Could you check a few things on this model? Use its own coordinates, in mm. A direction names the side the tool comes from. Give positions to 0.01 mm unless a question says otherwise; leave off trailing zeros. Order: outer loops, then holes, each group sorted by start corner. A loop starts at its lowest first (then second) coordinate and runs counter-clockwise, first axis right, second up.
(1) Imagine slicing it at A-A, the plane x = -46. Write out the boundary of the cut face in (y, z).
(2) If I drill on probe 1 along Z at (x, y) = (-12, -18.5); probe 2 along Z at (x, y) = (-46.5, -26.5); probe 3 along Y at (x, z) = (-13, -15), over which ranges is the centre line in solid material (lowest first)?
(3) Imagine slicing it at B-B, the plane y = 44. Write out the boundary of the cut face in (x, z).
(4) Imagine slicing it at C-C, the plane z = 3. Write out the boundary of the cut face in (x, y).
(5) Imagine slicing it at D-D, the plane y = -28. Write out the boundary of the cut face in (x, z).
(6) On a 3-axis mill with a long thin cutter (end or side, diameter ignored), from which of +Z, -Z, +X, -X, +Y, -Y can I reach the whole of each face in a straight line? I mean faces 1 (the flat face through (-5, -55, -6.604)), 2 (the flat face through (0, 0, 243.84)), 3 (the flat face through (9.6, 49.2, 0)). Say none if no direction works.
(7) Will these pins go through, and if not, where does the flat tip stop? pin 1 (8 mm diameter, centred on x = -14.5, z = 207.5, fed in from +Y); pin 2 (2 mm diameter, centred on x = -30, y = 31, fed in from +Z); pin 3 (23.5 mm diameter, centred on x = -7, y = -18.5, fed in from +Z).
from build123d import *

# Parameters (mm, degrees)
SKETCH1_R           = 49.9618
BOSS_EXTRUDE1_DEPTH = 78.74
SKETCH2_R           = 66.802
BOSS_EXTRUDE2_DEPTH = 6.604
SKETCH3_R           = 54.864
BOSS_EXTRUDE3_DEPTH = 17.78
SKETCH4_R           = 11.878006526
BOSS_EXTRUDE4_DEPTH = 12.7
BOSS_EXTRUDE5_DEPTH = 38.1
SKETCH7_R           = 39.497
BOSS_EXTRUDE6_DEPTH = 160.02
SKETCH8_R           = 6.058651835
BOSS_EXTRUDE7_DEPTH = 5.08


with BuildPart() as part:
    # Sketch1 → Boss-Extrude1 (new body)
    with BuildSketch(Plane.XY):
        Circle(SKETCH1_R)
    extrude(amount=BOSS_EXTRUDE1_DEPTH)

    # Sketch2 → Boss-Extrude2 (add)
    with BuildSketch(Plane(origin=(0, 0, 0), x_dir=(-1, 0, 0), z_dir=(0, 0, -1))):
        with Locations(Location((0, 0, 0), (0, 0, 180))):
            Circle(SKETCH2_R)
    extrude(amount=BOSS_EXTRUDE2_DEPTH)

    # Sketch3 → Boss-Extrude3 (add)
    with BuildSketch(Plane(origin=(0, 0, -6.604), x_dir=(-1, 0, 0), z_dir=(0, 0, -1))):
        Circle(SKETCH3_R)
    extrude(amount=BOSS_EXTRUDE3_DEPTH)

    # Sketch4 → Boss-Extrude4 (add)
    with BuildSketch(Plane(origin=(0, 0, -24.384), x_dir=(-1, 0, 0), z_dir=(0, 0, -1))):
        Circle(SKETCH4_R)
    extrude(amount=BOSS_EXTRUDE4_DEPTH)

    # Sketch5 → Boss-Extrude5 (add)
    with BuildSketch(Plane(origin=(0, 0, -37.084), x_dir=(-1, 0, 0), z_dir=(0, 0, -1))):
        Polygon((8.315334724, 0), (5.74575498, 1.866908963), (6.727247106, 4.887631119), (3.551071869, 4.887631119), (2.569579744, 7.908353274), (0, 6.041444312), (-2.569579744, 7.908353274), (-3.551071869, 4.887631119), (-6.727247106, 4.887631119), (-5.74575498, 1.866908963), (-8.315334724, 0), (-5.74575498, -1.866908963), (-6.727247106, -4.887631119), (-3.551071869, -4.887631119), (-2.569579744, -7.908353274), (0, -6.041444312), (2.569579744, -7.908353274), (3.551071869, -4.887631119), (6.727247106, -4.887631119), (5.74575498, -1.866908963), align=None)
    extrude(amount=BOSS_EXTRUDE5_DEPTH)

    # Sketch7 → Boss-Extrude6 (add)
    with BuildSketch(Plane.XY.offset(78.74)):
        Circle(SKETCH7_R)
    extrude(amount=BOSS_EXTRUDE6_DEPTH)

    # Sketch8 → Boss-Extrude7 (add)
    with BuildSketch(Plane.XY.offset(238.76)):
        Circle(SKETCH8_R)
    extrude(amount=BOSS_EXTRUDE7_DEPTH)


solid = part.part
Answer block:
1. outline: (-48.44, -6.6) - (-29.9, -6.6) - (-29.9, -24.38) - (29.9, -24.38) - (29.9, -6.6) - (48.44, -6.6) - (48.44, 0) - (19.5, 0) - (19.5, 78.74) - (-19.5, 78.74) - (-19.5, 0) - (-48.44, 0) - close
2. probe 1: z = -24.38 to 238.76
2. probe 2: z = -24.38 to 0
2. probe 3: y = -53.3 to 53.3
3. outline: (-50.26, -6.6) - (-32.77, -6.6) - (-32.77, -24.38) - (32.77, -24.38) - (32.77, -6.6) - (50.26, -6.6) - (50.26, 0) - (23.67, 0) - (23.67, 78.74) - (-23.67, 78.74) - (-23.67, 0) - (-50.26, 0) - close
4. outline: circle Ø99.92 at (0, 0)
5. outline: (-60.65, -6.6) - (-47.18, -6.6) - (-47.18, -24.38) - (47.18, -24.38) - (47.18, -6.6) - (60.65, -6.6) - (60.65, 0) - (41.38, 0) - (41.38, 78.74) - (27.86, 78.74) - (27.86, 238.76) - (-27.86, 238.76) - (-27.86, 78.74) - (-41.38, 78.74) - (-41.38, 0) - (-60.65, 0) - close
6. face 1: -Z
6. face 2: +Z, +X, -X, +Y, -Y
6. face 3: +Z
7. pin 1: stops at y = 38.08
7. pin 2: stops at z = 78.74
7. pin 3: stops at z = 238.76
